Autodesk Inventor part; units mm, degrees
ref_plane "YZ Plane" through (0, 0, 0) normal (1, 0, 0) x (0, 1, 0)
ref_plane "XZ Plane" through (0, 0, 0) normal (0, 1, 0) x (-1, 0, 0)
ref_plane "XY Plane" through (0, 0, 0) normal (0, 0, 1) x (1, 0, 0)
sketch "Sketch1" plane through (0, 0, 0) normal (0, 1, 0) x (-1, 0, 0)
  line L0 (-12.7, -19.05) -> (12.7, -19.05)
  line L1 (12.7, -19.05) -> (12.7, 19.05)
  line L2 (12.7, 19.05) -> (-12.7, 19.05)
  line L3 (-12.7, 19.05) -> (-12.7, -19.05)
  line L4 (-12.7, -19.05) -> (12.7, 19.05) construction
  line L5 (12.7, -19.05) -> (-12.7, 19.05) construction
  line L6 (12.7, 19.05) -> (0, 19.05)
  line L7 (0, 19.05) -> (0, -19.05)
  line L8 (0, -19.05) -> (12.7, -19.05)
  line L9 (12.7, -19.05) -> (12.7, 19.05)
  line L10 (0, 19.05) -> (-12.7, 6.35)
  line L11 (0, 19.05) -> (17.9605, 19.05) construction
  line L12 (0, -19.05) -> (-12.7, -6.35)
  line L13 (0, -19.05) -> (17.9605, -19.05) construction
  circle A0 centre (6.35, 0) radius 2.1828
  circle A1 centre (-6.35, 0) radius 2.1828
  circle A2 centre (6.35, 12.7) radius 2.1828
  circle A3 centre (6.35, -12.7) radius 2.1828
  point P0 (0, 0)
  point P1 (0, 0)
  point P2 (8.9803, -19.05)
  dimension "d0" = 25.4
  dimension "d1" = 38.1
  dimension "d2" = 135
  dimension "d3" = 135
  dimension "d4" = 4.3656
  dimension "d5" = 4.3656
  dimension "d6" = 4.3656
  dimension "d7" = 4.3656
  dimension "d10" = 12.7
  dimension "d11" = 6.35
  dimension "d12" = 19.05
  dimension "d13" = 19.05
extrude "Extrusion1" add sketch "Sketch1" along normal blind 1.5875 contours L7 L2 L1 L0 | L12 L3 L10 L7
properties part number "bracket1"
The model under review builds one solid part; all positions refer to its coordinate system, in mm. Round coordinates to 2 decimals unless told otherwise and drop trailing zeros. Loops run counter-clockwise (first coordinate to the right, second up) from the corner with the lowest first, then second, coordinate; pieces in that order, holes last. Notation, with made-up numbers: M 33.5,47 L 72.5,47 A20 ccw 72.5,85 Z; hole C 61.25,-39.75 d10. An arc over 180 degrees is marked long. Put each result on its own line as item: value.
Q1. Consider section A-A, the plane x = 6.35. Give the boundary of the cut face in (y, z).
Result set:
outline: M 0,-12.7 L 1.59,-12.7 L 1.59,-2.18 L 0,-2.18 Z; M 0,2.18 L 1.59,2.18 L 1.59,12.7 L 0,12.7 Z
Q2. Consider section C-C, the plane y = 0.35. Give the boundary of the cut face in (x, z), then the cut area to 3 significant figures.
Result set:
outline: M -12.7,-19.05 L 0,-19.05 L 12.7,-6.35 L 12.7,6.35 L 0,19.05 L -12.7,19.05 Z; hole C -6.35,-12.7 d4.37; hole C -6.35,0 d4.37; hole C -6.35,12.7 d4.37; hole C 6.35,0 d4.37
area: 747 mm²
Q3. To check wall thickness, follow L1, parallel to Z at x = -6.35, y = 1.25; L2, parallel to Z at x = -5, y = 1.4; L3, parallel to Z at x = 6.35, y = 0.6. State the ranges of each line that lie inside material, in increasing order.
Result set:
L1: z = -19.05 to -14.88, -10.52 to -2.18, 2.18 to 10.52, 14.88 to 19.05
L2: z = -19.05 to -14.42, -10.98 to -1.72, 1.72 to 10.98, 14.42 to 19.05
L3: z = -12.7 to -2.18, 2.18 to 12.7
Q4. Consider section D-D, the plane z = -12.7. Give the boundary of the cut face in (x, y), then the cut area to 3 significant figures.
Result set:
outline: M -12.7,0 L -8.53,0 L -8.53,1.59 L -12.7,1.59 Z; M -4.17,0 L 6.35,0 L 6.35,1.59 L -4.17,1.59 Z
area: 23.3 mm²
Q5. Consider section B-B, the plane z = 0. Give the boundary of the cut face in (x, y), then the cut area to 3 significant figures.
Result set:
outline: M -12.7,0 L -8.53,0 L -8.53,1.59 L -12.7,1.59 Z; M -4.17,0 L 4.17,0 L 4.17,1.59 L -4.17,1.59 Z; M 8.53,0 L 12.7,0 L 12.7,1.59 L 8.53,1.59 Z
area: 26.5 mm²
Q6. Mouldability with a two-part tool opening along Z and no side actions: class faces 1 (the flat face through (6.26, 0.78, 12.79)), 2 (the flat face through (6.26, 0.78, -12.79)), 3 (the cylindrical face through (-6.066, 0.783, 10.536)), 4 (the flat face through (12.7, 1, 0)) as released by +Z, released by -Z, zero draft, split by the parting line, or undercut.
Result set:
face 1: released by +Z
face 2: released by -Z
face 3: undercut
face 4: zero draft
